```python
from build123d import *

# Parameters (mm, degrees)
SKETCH33_R          = 28.6
SKETCH33_R_2        = 27.6
BOSS_EXTRUDE7_DEPTH = 5
BOSS_EXTRUDE8_START = 22
SKETCH33_11_R       = 20
BOSS_EXTRUDE8_DEPTH = 1
SKETCH33_12_R       = 27.6
SKETCH33_12_R_2     = 26
BOSS_EXTRUDE9_DEPTH = 2
SKETCH33_14_R       = 26
SKETCH33_14_R_2     = 20
CUT_EXTRUDE1_DEPTH  = 4.5
FILLET1_R           = 0.5
FILLET3_R           = 5


with BuildPart() as part:
    # Sketch33 → Boss-Extrude7 (new body)
    with BuildSketch(Plane(origin=(0, 0, 0), x_dir=(1, 0, 0), z_dir=(0, 1, 0))):
        with Locations(Location((0, 0, 0), (0, 0, 270))):
            Circle(SKETCH33_R)
        with Locations(Location((0, 0, 0), (0, 0, 270))):
            Circle(SKETCH33_R_2, mode=Mode.SUBTRACT)
    extrude(amount=-BOSS_EXTRUDE7_DEPTH)



with BuildPart() as body_2:
    # Sketch33<11> → Boss-Extrude8 (new body)
    with BuildSketch(Plane(origin=(0, 0, 0), x_dir=(1, 0, 0), z_dir=(0, 1, 0)).offset(BOSS_EXTRUDE8_START)):
        with Locations(Location((0, 0, 0), (0, 0, 270))):
            Circle(SKETCH33_11_R)
    extrude(amount=BOSS_EXTRUDE8_DEPTH)


with BuildPart() as body_3:
    # Sketch33<12> → Boss-Extrude9 (new body)
    with BuildSketch(Plane(origin=(0, 0, 0), x_dir=(1, 0, 0), z_dir=(0, 1, 0))):
        with Locations(Location((0, 0, 0), (0, 0, 270))):
            Circle(SKETCH33_12_R)
        with Locations(Location((0, 0, 0), (0, 0, 270))):
            Circle(SKETCH33_12_R_2, mode=Mode.SUBTRACT)
    extrude(amount=BOSS_EXTRUDE9_DEPTH)


with BuildPart() as part_1:
    add(part.part)

    add(body_3.part)  # loft5 joins it to this body
    # loft up to a face of the part (loft5)
    loft([Face(Wire([part_1.edges().sort_by_distance((20.848502744, 0, -19.57804723))[0]])), Face(Wire([part_1.edges().sort_by_distance((20.119534117, 2, -18.893500124))[0]]))])

    # Sketch33<14> → Cut-Extrude1 (cut)
    # profile 1 of 2: a face of its own
    with BuildSketch(Plane(origin=(0, 0, 0), x_dir=(1, 0, 0), z_dir=(0, 1, 0))):
        with Locations(Location((0, 0, 0), (0, 0, 270))):
            Circle(SKETCH33_14_R)
        with Locations(Location((0, 0, 0), (0, 0, 270))):
            Circle(SKETCH33_14_R_2, mode=Mode.SUBTRACT)
    # profile 2 of 2: a face of its own
    with BuildSketch(Plane(origin=(0, 0, 0), x_dir=(1, 0, 0), z_dir=(0, 1, 0))):
        with Locations(Location((0, 0, 0), (0, 0, 270))):
            Circle(SKETCH33_14_R_2)
    extrude(amount=CUT_EXTRUDE1_DEPTH, mode=Mode.SUBTRACT)


    add(body_2.part)  # loft6 joins it to this body
    # loft up to a face of the part (loft6)
    loft([Face(Wire([part_1.edges().sort_by_distance((20.119534117, 2, -18.893500124))[0]])), Face(Wire([part_1.edges().sort_by_distance((14.579372548, 23, -13.690942119))[0]]))])

    # Sketch35 → Cut-Revolve4 (revolve, cut)
    with BuildSketch(Plane.XY, mode=Mode.PRIVATE) as cut_revolve4_sk:
        Polygon((-26, 2), (-19, 22), (0, 22), (0, 2), align=None)
    revolve(cut_revolve4_sk.sketch.rotate(Axis((0, 22, 0), (0, -1, 0)), 270), axis=Axis((0, 22, 0), (0, -1, 0)), mode=Mode.SUBTRACT)

    # Fillet1
    fillet1_edges = [part_1.edges().sort_by_distance(p)[0] for p in [
        (0, -5, -28.6),
        (0, -5, -27.6),
    ]]
    fillet(fillet1_edges, radius=FILLET1_R - 0.0001)  # a hair under: the kernel refuses the full size

    # Fillet3
    fillet3_edges = [part_1.edges().sort_by_distance(p)[0] for p in [
        (0, 0, -28.6),
    ]]
    fillet(fillet3_edges, radius=FILLET3_R)


solid = part_1.part
```
Geometry check sheet. Reference: the model listing, model coordinates, mm. A direction names the side the tool comes from. Give positions to 0.01 mm unless a question says otherwise; leave off trailing zeros. Order: outer loops, then holes, each group sorted by start corner. A loop starts at its lowest first (then second) coordinate and runs counter-clockwise, first axis right, second up. Notation, with made-up numbers: (-1.75, 0) -> (37.25, 0) arc R34 cw to (37.25, 32) -> close; hole circle Ø11 at (-19, 70). An arc over 180 degrees is marked (long way). Write each question's results on one line, items separated by ' | '. Start each with the question number.
(1) Access from +Z, -Z, +X, -X, +Y, -Y to the whole of each face (thin tool, end or side, straight path). Record for faces 1 (the face through (-18, 0, -19)), 2 (the face through (8.59, -2.82, 27.28)).
(2) Sectioned sample at A-A (y = 14). Enter the section's corners in (x, z), plus the area to 3 significant figures.
(3) Mould release check, pull along X, two halves, no side actions. Record for faces 3 (the face through (-20.709, 19.647, -4.599)), 4 (the face through (0, 23, 0)), 5 (the face through (18.7, -2.2, -20.3)): pulls with the +X half, pulls with the -X half, needs draft (parallel to the pull), parting line crosses it, or undercut.
(4) Scan lines: line 1 (X direction, y = -2.05, z = 0); line 2 (Y direction, x = -10.5, z = -1); line 3 (X direction, y = 0.85, z = 0). Record each from-to range of solid material in increasing order.
(5) Gauge pin test, flat ends, axial feed: P1, Ø8, axis at x = -13, y = 16, coming from the +Z side; P2, Ø3, axis at y = 8.5, z = -9.5, coming from the +X side; P3, Ø3, axis at x = -15, y = 9.5, coming from the -Z side. Record the tip position at first contact, or that the pin passes through.
Answer below:
1) face 1: -Y | face 2: +Y, -Y
2) outline: circle Ø46.51 at (0, 0); hole circle Ø43.6 at (0, 0) | area: 206 mm2
3) face 3: parting line crosses it | face 4: needs draft | face 5: undercut
4) line 1: -28.6 to -27.6, 27.6 to 28.6 | line 2: 22 to 23 | line 3: -28.17 to -26, 26 to 28.17
5) P1: z = 21.26 | P2: x = 24.2 | P3: z = -21.1
